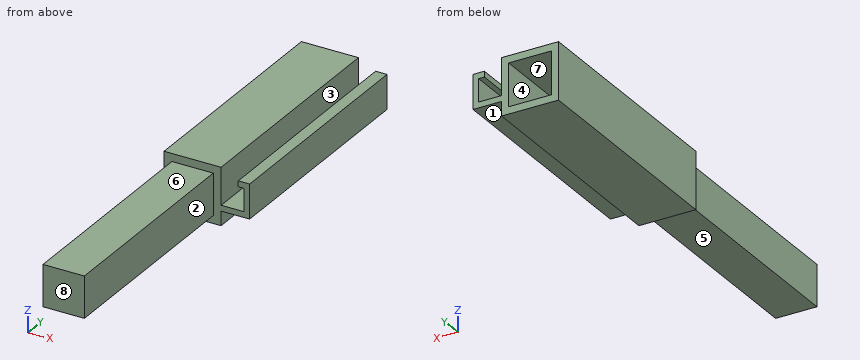
Autodesk Inventor part; units mm, degrees
ref_plane "YZ Plane" through (0, 0, 0) normal (1, 0, 0) x (0, 1, 0)
ref_plane "XZ Plane" through (0, 0, 0) normal (0, 1, 0) x (-1, 0, 0)
ref_plane "XY Plane" through (0, 0, 0) normal (0, 0, 1) x (1, 0, 0)
sketch "Sketch1" plane through (0, 0, 0) normal (0, 1, 0) x (-1, 0, 0)
  line L0 (-7.25, 7.25) -> (7.25, 7.25)
  line L1 (7.25, 7.25) -> (7.25, -7.25)
  line L2 (7.25, -7.25) -> (-7.25, -7.25)
  line L3 (-7.25, -7.25) -> (-7.25, 7.25)
  line L4 (-7.25, 7.25) -> (7.25, -7.25) construction
  line L5 (7.25, 7.25) -> (-7.25, -7.25) construction
  point P0 (0, 0)
  dimension "d0" = 14.5
  dimension "d1" = 14.5
extrude "Extrusion1" add sketch "Sketch1" along normal blind 76.2
sketch "Sketch2" plane through (0, 76.2, 0) normal (0, 1, 0) x (1, 0, 0)
  line L0 (10, -10) -> (-10, -10)
  line L1 (-10, -10) -> (-10, 10)
  line L2 (-10, 10) -> (10, 10)
  line L3 (10, 10) -> (10, -10)
  line L4 (10, -10) -> (-10, 10) construction
  line L5 (-10, -10) -> (10, 10) construction
  point P0 (0, 0)
  dimension "d4" = 20
  dimension "d5" = 20
extrude "Extrusion2" add sketch "Sketch2" along normal blind 5
sketch "Sketch3" plane through (0, 81.2, 0) normal (0, 1, 0) x (1, 0, 0)
  line L0 (7.5, -7.5) -> (-7.5, -7.5)
  line L1 (-7.5, -7.5) -> (-7.5, 7.5)
  line L2 (-7.5, 7.5) -> (7.5, 7.5)
  line L3 (7.5, 7.5) -> (7.5, -7.5)
  line L4 (7.5, -7.5) -> (-7.5, 7.5) construction
  line L5 (-7.5, -7.5) -> (7.5, 7.5) construction
  line L6 (10, -10) -> (-10, -10)
  line L7 (-10, -10) -> (-10, 10)
  line L8 (-10, 10) -> (10, 10)
  line L9 (10, 10) -> (10, -10)
  line L10 (10, -10) -> (-10, 10) construction
  line L11 (-10, -10) -> (10, 10) construction
  point P0 (0, 0)
  dimension "d8" = 15
  dimension "d9" = 15
extrude "Extrusion3" add sketch "Sketch3" along normal blind 76.2
sketch "Sketch4" plane through (10, 76.2, 10) normal (1, 0, 0) x (0, 0, -1)
  line L0 (20, 0) -> (20, 81.2)
  line L1 (15, 81.2) -> (15, 0)
  line L2 (0, 0) -> (20, 0)
  line L3 (15, 81.2) -> (13, 81.2)
  line L4 (17.5, 81.2) -> (2.5, 81.2)
  line L5 (13, 81.2) -> (13, 0)
  line L6 (13, 0) -> (15, 0)
  line L7 (20, 81.2) -> (0, 81.2)
  point P0 (10, -76.2)
  dimension "d12" = 2
extrude "Extrusion4" add sketch "Sketch4" along normal blind 10 contours L2 L5 L3 L1
sketch "Sketch5" plane through (10, 76.2, -3) normal (0, 0, 1) x (1, 0, 0)
  line L0 (0, 81.2) -> (10, 81.2)
  line L1 (10, 81.2) -> (8, 81.2)
  line L2 (8, 81.2) -> (8, 0)
  line L3 (8, 0) -> (10, 0)
  line L4 (10, 0) -> (10, 81.2)
  point P0 (-10, -76.2)
  dimension "d15" = 2
extrude "Extrusion5" add sketch "Sketch5" along normal blind 8
sketch "Sketch6" plane through (20, 76.2, 10) normal (1, 0, 0) x (0, 0, -1)
  line L0 (5, 81.2) -> (3, 81.2)
  line L1 (3, 81.2) -> (3, 0)
  line L2 (3, 0) -> (5, 0)
  line L3 (5, 0) -> (5, 81.2)
  point P0 (10, -76.2)
  dimension "d18" = 2
extrude "Extrusion6" add sketch "Sketch6" against normal blind 4
properties part number "CraneArmLink"
Model file for the job. Use its own axes, mm. Face numbers are marked on the shaded views. A direction names the side the tool comes from. Coordinates: 2 decimals unless noted, no trailing zeros. Write each loop counter-clockwise with the first axis right and the second up, starting at its lowest first coordinate (ties: lowest second). Pieces come first, ordered by that corner, then holes. Notation, with made-up numbers: (71.5, -25) - (113.5, -25) arc R25 cw to (113.5, -8) - close; hole circle Ø6 at (7.5, -7). An arc over 180 degrees is marked (long way). Use a Markdown table: item, result. Add a question column.
Item 1: Band-saw the part on D-D, the plane y = 35.5. Write the cut outline in (x, z).
Item 2: 3-axis set-ups, long thin cutter, end or side, ignore diameter. For the marked faces 1, 2, 3, 4 and 5: which of +Z, -Z, +X, -X, +Y, -Y reach the whole face in a straight line?
Item 3: Drill centre lines: line 1 along X through (y, z) = (91, 3.5); line 2 along Z through (x, y) = (-3.75, 141.5); line 3 along Y through (x, z) = (8, -4.5). Where is each one in solid material? Low to high.
Item 4: Drop flat-ended pins along their axis: pin 1 (3 mm diameter, centred on x = 15.5, y = 112.5, fed in from -Z); pin 2 (7 mm diameter, centred on y = 54, z = 2.5, fed in from +X); pin 3 (1 mm diameter, centred on x = 4, z = -5.5, fed in from +Y). Give the stop position or say it passes through.
Item 5: Band-saw the part on B-B, the plane y = 125. Write the cut outline in (x, z), and give its area (3 significant figures).
Item 6: Band-saw the part on A-A, the plane z = 2.25. Write the cut outline in (x, y), and give its area (3 significant figures).
Item 7: Band-saw the part on C-C, the plane x = 0.25. Write the cut outline in (y, z), and give its area (3 significant figures).
Item 8: Two-plate mould, pull along Z, no slides. Class the marked faces 6, 7 and 8: pulls with the +Z half, pulls with the -Z half, needs draft (parallel to the pull), parting line crosses it, or undercut.
A:
| question | item | result |
|---|---|---|
| 1 | outline | (-7.25, -7.25) - (7.25, -7.25) - (7.25, 7.25) - (-7.25, 7.25) - close |
| 2 | face 1 | -Z, +X, +Y, -Y |
| 2 | face 2 | +Z, -Z, +X, -Y |
| 2 | face 3 | +Z, +Y, -Y |
| 2 | face 4 | +Y |
| 2 | face 5 | -Z, +X, -X, -Y |
| 3 | line 1 | x = -10 to -7.5, 7.5 to 10, 18 to 20 |
| 3 | line 2 | z = -10 to -7.5, 7.5 to 10 |
| 3 | line 3 | y = 76.2 to 157.4 |
| 4 | pin 1 | stops at z = -5 |
| 4 | pin 2 | stops at x = 7.25 |
| 4 | pin 3 | stops at y = 81.2 |
| 5 | outline | (-10, -10) - (10, -10) - (10, -5) - (20, -5) - (20, 7) - (16, 7) - (16, 5) - (18, 5) - (18, -3) - (10, -3) - (10, 10) - (-10, 10) - close; hole (-7.5, -7.5) - (7.5, -7.5) - (7.5, 7.5) - (-7.5, 7.5) - close |
| 5 | area | 219 mm² |
| 6 | outline | (-10, 76.2) - (-7.25, 76.2) - (-7.25, 0) - (7.25, 0) - (7.25, 76.2) - (10, 76.2) - (10, 157.4) - (7.5, 157.4) - (7.5, 81.2) - (-7.5, 81.2) - (-7.5, 157.4) - (-10, 157.4) - close; (18, 76.2) - (20, 76.2) - (20, 157.4) - (18, 157.4) - close |
| 6 | area | 1,750 mm² |
| 7 | outline | (0, -7.25) - (76.2, -7.25) - (76.2, -10) - (157.4, -10) - (157.4, -7.5) - (81.2, -7.5) - (81.2, 7.5) - (157.4, 7.5) - (157.4, 10) - (76.2, 10) - (76.2, 7.25) - (0, 7.25) - close |
| 7 | area | 1,590 mm² |
| 8 | face 6 | pulls with the +Z half |
| 8 | face 7 | undercut |
| 8 | face 8 | needs draft |
